For this review, take the finished solid that the model builds, in its own axes (mm). Face numbers are marked on the shaded views. A direction names the side the tool comes from. Give positions to 0.01 mm unless a question says otherwise; leave off trailing zeros. Write each loop counter-clockwise with the first axis right and the second up, starting at its lowest first coordinate (ties: lowest second). Pieces come first, ordered by that corner, then holes.
Q1. We need section C-C (y = -1.7). Write out the cut boundary in (x, z), then the cut area to 3 significant figures.
Q2. For line 1 (X direction, y = 2.2, z = 0); line 2 (X direction, y = -1, z = 0); line 3 (Y direction, x = 17.5, z = -4), list the stretches that pass through material, from the lowest coordinate up.
Q3. We need section D-D (x = 7). Write out the cut boundary in (y, z).
Q4. We need section B-B (z = 1.5). Write out the cut boundary in (x, y), then the cut area to 3 significant figures.
Q5. Insertion check: P1, Ø2, axis at x = 0, z = 0, coming from the +Y side; P2, Ø1.5, axis at x = 23.5, z = -4, coming from the -Y side; P3, Ø1.6, axis at x = 0, z = -1, coming from the -Y side. Each pin has a flat end and moves straight along its axis. Give the tip position at first contact, or say it passes through.
Q6. We need section A-A (z = 0). Write out the cut boundary in (x, y).
Q7. Machinability: for the marked faces 1 and 2, which of the approach directions +Z, -Z, +X, -X, +Y, -Y give a long, thin tool a straight path to every point of the face, cutting with its end or side? Answer none if there is none.
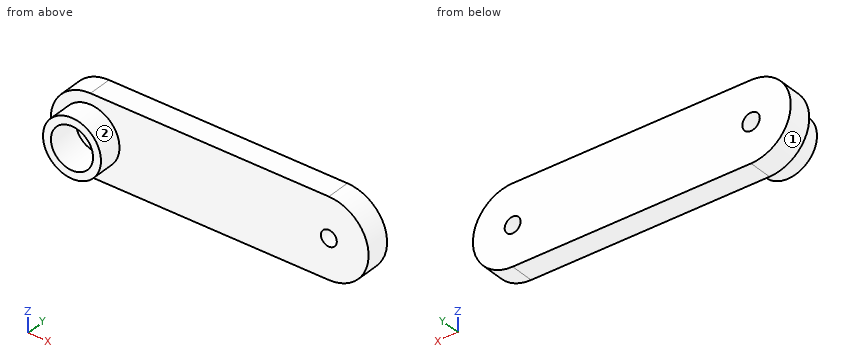
```python
from build123d import *

# Parameters (mm, degrees)
BOSS_EXTRUDE1_DEPTH = 3
SKETCH2_R           = 3.65
BOSS_EXTRUDE2_DEPTH = 3
SKETCH3_R           = 1.1
CUT_EXTRUDE1_DEPTH  = 6
SKETCH5_R           = 2.65
CUT_EXTRUDE2_DEPTH  = 4
SKETCH7_R           = 1
CUT_EXTRUDE4_DEPTH  = 3


with BuildPart() as part:
    # Sketch1 → Boss-Extrude1 (new body)
    with BuildSketch(Plane(origin=(0, 0, 0), x_dir=(1, 0, 0), z_dir=(0, 1, 0))):
        with BuildLine():
            Line((0, 5), (30, 5))
            ThreePointArc((30, 5), (35, 0), (30, -5))
            Line((30, -5), (0, -5))
            ThreePointArc((0, -5), (-5, 0), (0, 5))
        make_face()
    extrude(amount=BOSS_EXTRUDE1_DEPTH)

    # Sketch2 → Boss-Extrude2 (add)
    with BuildSketch(Plane.XZ):
        with Locations(Location((0, 0, 0), (0, 0, 90))):
            Circle(SKETCH2_R)
    extrude(amount=BOSS_EXTRUDE2_DEPTH)

    # Sketch3 → Cut-Extrude1 (cut)
    with BuildSketch(Plane.XZ.offset(3)):
        with Locations(Location((0, 0, 0), (0, 0, 270))):
            Circle(SKETCH3_R)
    extrude(amount=-CUT_EXTRUDE1_DEPTH, mode=Mode.SUBTRACT)

    # Sketch5 → Cut-Extrude2 (cut)
    with BuildSketch(Plane.XZ.offset(3)):
        with Locations(Location((0, 0, 0), (0, 0, 270))):
            Circle(SKETCH5_R)
    extrude(amount=-CUT_EXTRUDE2_DEPTH, mode=Mode.SUBTRACT)

    # Sketch7 → Cut-Extrude4 (cut)
    with BuildSketch(Plane(origin=(0, 3, 0), x_dir=(1, 0, 0), z_dir=(0, 1, 0))):
        with Locations(Location((30, 0, 0), (0, 0, 270))):
            Circle(SKETCH7_R)
    extrude(amount=-CUT_EXTRUDE4_DEPTH, mode=Mode.SUBTRACT)


solid = part.part
```
Computed:
1. outline: circle Ø7.3 at (0, 0); hole circle Ø5.3 at (0, 0)
1. area: 19.8 mm2
2. line 1: x = -5 to -1.1, 1.1 to 29, 31 to 35
2. line 2: x = -3.65 to -2.65, 2.65 to 3.65
2. line 3: y = 0 to 3
3. outline: (0, -5) - (3, -5) - (3, 5) - (0, 5) - close
4. outline: (-4.77, 0) - (-3.33, 0) - (-3.33, -3) - (-2.18, -3) - (-2.18, 1) - (2.18, 1) - (2.18, -3) - (3.33, -3) - (3.33, 0) - (34.77, 0) - (34.77, 3) - (-4.77, 3) - close
4. area: 121 mm2
5. P1: passes through
5. P2: stops at y = 0
5. P3: stops at y = 1
6. outline: (-5, 0) - (-3.65, 0) - (-3.65, -3) - (-2.65, -3) - (-2.65, 1) - (-1.1, 1) - (-1.1, 3) - (-5, 3) - close; (1.1, 1) - (2.65, 1) - (2.65, -3) - (3.65, -3) - (3.65, 0) - (29, 0) - (29, 3) - (1.1, 3) - close; (31, 0) - (35, 0) - (35, 3) - (31, 3) - close
7. face 1: -X, +Y, -Y
7. face 2: -Y
